Could you check a few things on this drawing? It's one solid part, dimensions in mm from its lowest x, y, z. A direction names the side the tool comes from. Round coordinates to 2 decimals unless told otherwise and drop trailing zeros. Write each loop counter-clockwise with the first axis right and the second up, starting at its lowest first coordinate (ties: lowest second). Pieces come first, ordered by that corner, then holes. Notation, with made-up numbers: (31.5, 67) -> (70.5, 67) arc R23 ccw to (70.5, 80) -> close; hole circle Ø10 at (-25, 67.5). An arc over 180 degrees is marked (long way). Put each result on its own line as item: value. Start each with the question number.
1) I want a section at B-B, the plane y = 25. List the corners of the cut face in (x, z) for me, then the cut area to 3 significant figures.
2) We'd pull the mould along Y, two halves only. Please class the marked faces 6, 7 and 8: released by +Y, released by -Y, zero draft, split by the parting line, or undercut.
3) I want a section at C-C, the plane y = 4. List the corners of the cut face in (x, z) for me.
4) If I drill on line 1 along Z through (x, y) = (9.6, 25); line 2 along Y through (x, z) = (64.95, 3); line 3 along Y through (x, z) = (7, 3.2), over which ranges is the centre line in solid material (lowest first)? Write a range as [from, to].
5) I want a section at A-A, the plane x = 9. List the corners of the cut face in (y, z) for me, then the cut area to 3 significant figures.
6) Will these pins go through, and if not, where does the flat tip stop? P1, Ø3, axis at y = 43.5, z = 2, coming from the +X side; P2, Ø2, axis at y = 41.5, z = 4.5, coming from the -X side; P3, Ø2.5, axis at y = 25, z = 3, coming from the +X side.
7) Which directions (+Z, -Z, +X, -X, +Y, -Y) give clear straight access to the entire face, cutting with the end or side of a thin tool? Please do the marked faces 1, 2, 3, 4 and 5.
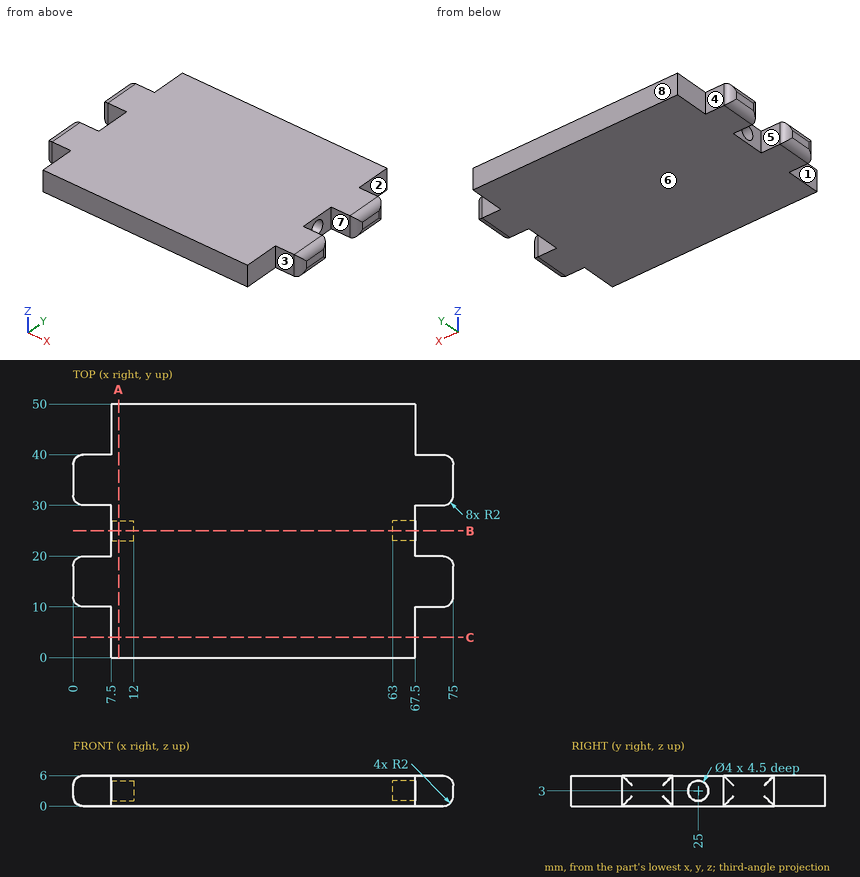
Findings:
1. outline: (7.5, 0) -> (67.5, 0) -> (67.5, 1) -> (63, 1) -> (63, 5) -> (67.5, 5) -> (67.5, 6) -> (7.5, 6) -> (7.5, 5) -> (12, 5) -> (12, 1) -> (7.5, 1) -> close
1. area: 324 mm2
2. face 6: zero draft
2. face 7: undercut
2. face 8: released by +Y
3. outline: (7.5, 0) -> (67.5, 0) -> (67.5, 6) -> (7.5, 6) -> close
4. line 1: z = [0, 1], [5, 6]
4. line 2: y = [0, 23], [27, 50]
4. line 3: y = [10, 20], [30, 40]
5. outline: (0, 0) -> (50, 0) -> (50, 6) -> (0, 6) -> close; hole circle Ø4 at (25, 3)
5. area: 287 mm2
6. P1: stops at x = 67.5
6. P2: stops at x = 7.5
6. P3: stops at x = 63
7. face 1: +Z, -Z, -X, -Y
7. face 2: +Z, -Z, +X, +Y
7. face 3: +Z, -Z, +X, -Y
7. face 4: +Z, -Z, -X, +Y
7. face 5: +Z, -Z, -X
